Design review of the part shown in the three views and the two pictorial views. Dimensions are in mm from the part's minimum x, y and z. Coordinates: 2 decimals unless noted, no trailing zeros. Loops run counter-clockwise (first coordinate to the right, second up) from the corner with the lowest first, then second, coordinate; pieces in that order, holes last. Notation, with made-up numbers: M -1,63.5 L 18,63.5 A19 ccw 18,82.5 Z; hole C 35.25,74.5 d1. An arc over 180 degrees is marked long. Put each result on its own line as item: value. Start each with the question number.
(1) The part is to be moulded in two halves that separate along Y. For the marked faces 1, 2 and 3, say which applies: +Y half, -Y half, draft (parallel to the pull), parting line (faces both ways), or undercut.
(2) For probe 1 along Z at (x, y) = (30.5, 85); probe 2 along Y at (x, z) = (26.5, 27) (1 decimal); probe 3 along Y at (x, z) = (10, 11) (1 decimal), list the stretches that pass through material, from the lowest coordinate up. Write a range as [from, to].
(3) Take a section at D-D, the plane z = 13.5. Give the boundary of the cut face in (x, y).
(4) Take a section at C-C, the plane x = 17.5. Count the separate pieces of the cut face and the enclosed holes in it, then the cut area to 3 significant figures.
(5) Take a section at B-B, the plane y = 50.8. Give the boundary of the cut face in (x, z), then the cut area to 3 significant figures.
(6) Take a section at A-A, the plane z = 19.05. Give the boundary of the cut face in (x, y).
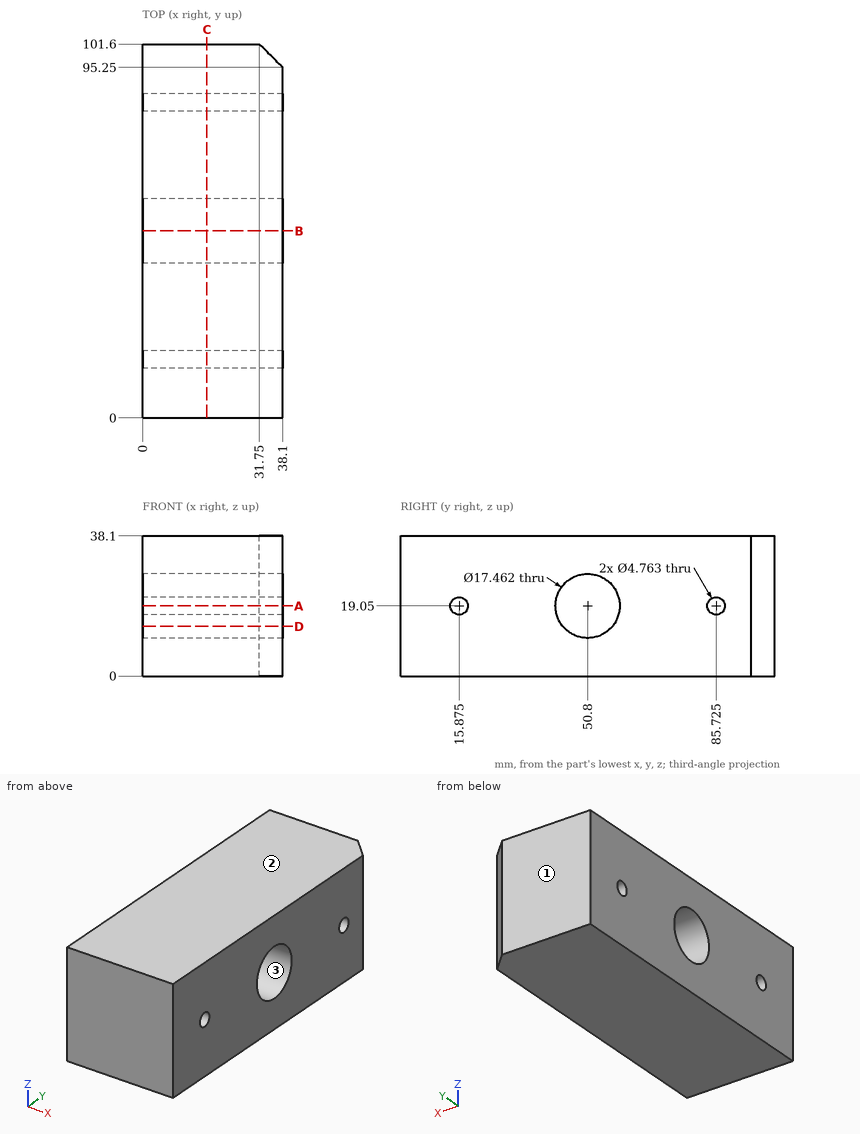
Computed values:
1. face 1: +Y half
1. face 2: draft
1. face 3: undercut
2. probe 1: z = [0, 16.78], [21.32, 38.1]
2. probe 2: y = [0, 47.2], [54.4, 101.6]
2. probe 3: y = [0, 47.4], [54.2, 101.6]
3. outline: M 0,0 L 38.1,0 L 38.1,44.06 L 0,44.06 Z; M 0,57.54 L 38.1,57.54 L 38.1,95.25 L 31.75,101.6 L 0,101.6 Z
4. separate pieces: 1
4. enclosed holes: 3
4. area: 3,600 mm^2
5. outline: M 0,0 L 38.1,0 L 38.1,10.32 L 0,10.32 Z; M 0,27.78 L 38.1,27.78 L 38.1,38.1 L 0,38.1 Z
5. area: 786 mm^2
6. outline: M 0,0 L 38.1,0 L 38.1,13.49 L 0,13.49 Z; M 0,18.26 L 38.1,18.26 L 38.1,42.07 L 0,42.07 Z; M 0,59.53 L 38.1,59.53 L 38.1,83.34 L 0,83.34 Z; M 0,88.11 L 38.1,88.11 L 38.1,95.25 L 31.75,101.6 L 0,101.6 Z
